Check sheet for the modelled part. Datum: model origin and axes. Units: mm. Face numbers are marked on the shaded views. A direction names the side the tool comes from. Round coordinates to 2 decimals unless told otherwise and drop trailing zeros. Order: outer loops, then holes, each group sorted by start corner. A loop starts at its lowest first (then second) coordinate and runs counter-clockwise, first axis right, second up.
(1) Sectioned sample at C-C, the plane x = -41. Enter the section's corners in (y, z), and give its area (3 significant figures).
(2) Tool access check on the marked faces 4 and 5. Record the directions out of +Z, -Z, +X, -X, +Y, -Y that give a thin tool (end or side, any length) a straight path to the whole face; none if there is none.
(3) Mould release check, pull along Y, two halves, no side actions. Record for the marked faces 1, 2 and 3: released by +Y, released by -Y, zero draft, split by the parting line, or undercut.
(4) Thickness scan on probe 1 along X at (y, z) = (36, -15.75); probe 2 along Y at (x, z) = (-42, -1.75); probe 3 along Y at (x, z) = (-47, -25.5). Record the ranges inside material, lowest first.
(5) Sectioned sample at B-B, the plane z = -13.75. Enter the section's corners in (x, y), and give its area (3 significant figures).
(6) Depth check by flat-ended pin: pin 1 (4.5 mm diameter, centred on x = -50, z = -15, fed in from +Y); pin 2 (1.5 mm diameter, centred on x = -24, z = -9, fed in from +Y); pin 3 (4 mm diameter, centred on x = -52, y = 86.5, fed in from +Z). Enter the tip coordinate at first touch or a pass-through.
(7) Sectioned sample at A-A, the plane x = -50. Enter the section's corners in (y, z), and give its area (3 significant figures).
(8) Sectioned sample at D-D, the plane y = 78. Enter the section's corners in (x, z).
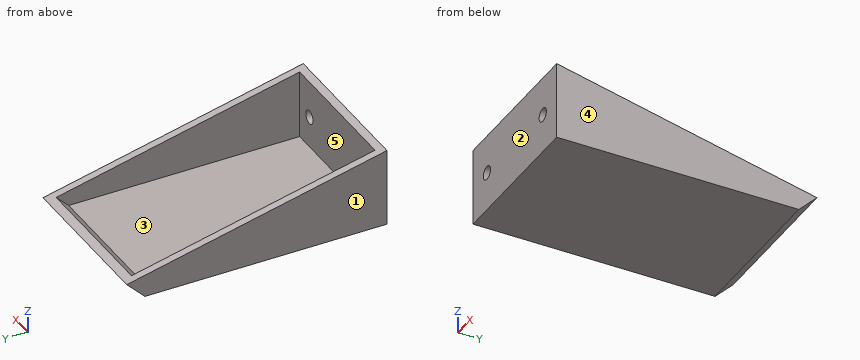
Autodesk Inventor part; units mm, degrees
ref_plane "YZ Plane" through (0, 0, 0) normal (1, 0, 0) x (0, 1, 0)
ref_plane "XZ Plane" through (0, 0, 0) normal (0, 1, 0) x (-1, 0, 0)
ref_plane "XY Plane" through (0, 0, 0) normal (0, 0, 1) x (1, 0, 0)
sketch "Sketch4" plane through (0, 0, 0) normal (0, 1, 0) x (-1, 0, 0)
  line L0 (0, 0) -> (60, 0)
  line L1 (60, 0) -> (60, -30)
  line L2 (60, -30) -> (0, -30)
  line L3 (0, -30) -> (0, 0)
  dimension "d15" = 60
  dimension "d16" = 30
extrude "Extrusion4" add sketch "Sketch4" along normal blind 100
chamfer "Chamfer1" distance 7 angle 45 1 edges at (-30, 100, -30)
sketch "Sketch6" plane through (0, 0, 0) normal (1, 0, 0) x (0, 0, -1)
  line L0 (30, 0) -> (30, 93)
  line L1 (0, 0) -> (0, 100)
  line L2 (30, 0) -> (0, 0)
  line L3 (0, 0) -> (0, 100)
  line L4 (0, 100) -> (30, 100)
  line L5 (30, 100) -> (30, 0)
  line L6 (0, 0) -> (23.0011, 100)
extrude "Extrusion5" cut sketch "Sketch6" against normal blind 100 contours L1 L4 L6
shell "Shell2" thickness 3 removed faces 1 at (-40, 66.6661, -15.3339)
sketch "Sketch8" plane through (0, 0, 0) normal (0, -1, 0) x (1, 0, 0)
  line L0 (0, -30) -> (-60, -30)
  line L1 (0, 0) -> (-60, 0)
  line L2 (-60, 0) -> (-60, -30)
  line L3 (-60, -30) -> (0, -30)
  line L4 (0, -30) -> (0, 0)
  line L5 (0, -23.0009) -> (0, 0)
  line L6 (0, 0) -> (0, -15)
  line L7 (0, -15) -> (-60, -15) construction
  line L8 (-30, 0) -> (-30, -30) construction
  line L9 (-30, -15) -> (-10, -15) construction
  circle A0 centre (-10, -15) radius 2.6
  line L10 (-30, -15) -> (-50, -15) construction
  circle A1 centre (-50, -15) radius 2.6
  dimension "d26" = 15
  dimension "d27" = 20
  dimension "d28" = 5.2
extrude "Extrusion6" cut sketch "Sketch8" against normal blind 20 contours A0 | A1
properties part number "Claw"
Derived:
1. outline: (0, -30) - (93, -30) - (100, -23) - (96.55, -22.21) - (91.76, -27) - (3, -27) - (3, -0.69) - (0, 0) - close
1. area: 382 mm2
2. face 4: +Z, -Z, +X, +Y, -Y
2. face 5: +Z
3. face 1: zero draft
3. face 2: released by -Y
3. face 3: undercut
4. probe 1: x = -60 to -57, -3 to 0
4. probe 2: y = 0 to 3
4. probe 3: y = 0 to 3, 93.26 to 97.5
5. outline: (-60, 0) - (-52.28, 0) - (-52.28, 3) - (-57, 3) - (-57, 59.78) - (-60, 59.78) - close; (-47.72, 0) - (-12.28, 0) - (-12.28, 3) - (-47.72, 3) - close; (-7.72, 0) - (0, 0) - (0, 59.78) - (-3, 59.78) - (-3, 3) - (-7.72, 3) - close
5. area: 493 mm2
6. pin 1: passes through
6. pin 2: stops at y = 3
6. pin 3: stops at z = -27
7. outline: (0, -30) - (93, -30) - (100, -23) - (96.55, -22.21) - (91.76, -27) - (3, -27) - (3, -17.6) - (0, -17.6) - close; (0, -12.4) - (3, -12.4) - (3, -0.69) - (0, 0) - close
7. area: 367 mm2
8. outline: (-60, -30) - (0, -30) - (0, -17.94) - (-3, -17.94) - (-3, -27) - (-57, -27) - (-57, -17.94) - (-60, -17.94) - close
